```python
from build123d import *

# Parameters (mm, degrees)
SKETCH_1_R      = 1.5
SKETCH_1_W      = 15
SKETCH_1_H      = 18
SKETCH_1_H_2    = 3
EXTRUDE_1_DEPTH = 3
FILLET_1_R      = 5


with BuildPart() as part:
    # 草图1 → 凸台-拉伸1 (new body)
    with BuildSketch(Plane.XY):
        with BuildLine():
            Line((0, 0), (0, 67))
            Line((0, 67), (20, 67))
            Line((20, 67), (22.897896607, 50.56521166))
            ThreePointArc((22.897896607, 50.56521166), (24.147168803, 48.042864005), (26.561036073, 46.595050647))
            ThreePointArc((26.561036073, 46.595050647), (37.908605389, 40.597944156), (45.388192925, 30.167777045))
            ThreePointArc((45.388192925, 30.167777045), (46.877900379, 28.176180142), (49.14284363, 27.148698467))
            Line((49.14284363, 27.148698467), (67, 24))
            Line((67, 24), (67, 0))
            Line((67, 0), (0, 0))
        make_face()
        with Locations((12, 62)):
            Circle(SKETCH_1_R, mode=Mode.SUBTRACT)
        with Locations((12, 42)):
            Circle(SKETCH_1_R, mode=Mode.SUBTRACT)
        with Locations((12, 22)):
            Circle(SKETCH_1_R, mode=Mode.SUBTRACT)
        with Locations(Location((62, 12, 0), (0, 0, 180))):
            Circle(SKETCH_1_R, mode=Mode.SUBTRACT)
        with Locations(Location((42, 12, 0), (0, 0, 180))):
            Circle(SKETCH_1_R, mode=Mode.SUBTRACT)
        with Locations(Location((22, 12, 0), (0, 0, 180))):
            Circle(SKETCH_1_R, mode=Mode.SUBTRACT)
        with Locations((27, 28.5)):
            Rectangle(SKETCH_1_W, SKETCH_1_H, mode=Mode.SUBTRACT)
        with Locations((52, 21)):
            Rectangle(SKETCH_1_W, SKETCH_1_H_2, mode=Mode.SUBTRACT)
    extrude(amount=EXTRUDE_1_DEPTH)

    # 圆角1
    fillet_1_edges = [part.edges().sort_by_distance(p)[0] for p in [
        (0, 0, 1.5),
        (0, 67, 1.5),
        (20, 67, 1.5),
        (67, 24, 1.5),
        (67, 0, 1.5),
    ]]
    fillet(fillet_1_edges, radius=FILLET_1_R)


solid = part.part
```
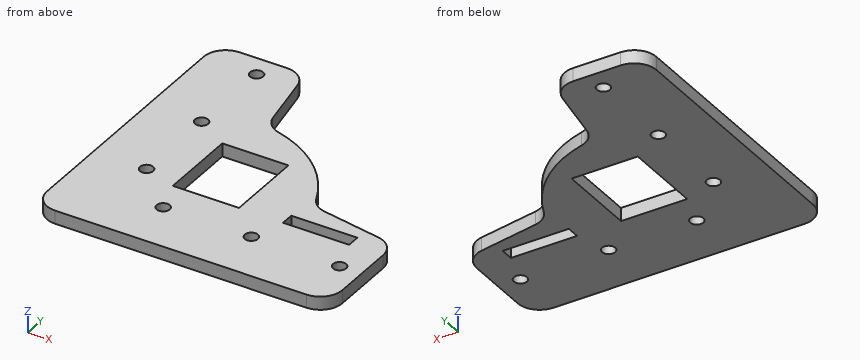
Design review of the part built by this model. Coordinates are the model's own, in mm. Give positions to 0.01 mm unless a question says otherwise; leave off trailing zeros. Order: outer loops, then holes, each group sorted by start corner. A loop starts at its lowest first (then second) coordinate and runs counter-clockwise, first axis right, second up. Notation, with made-up numbers: (77.5, 38.5) - (91.5, 38.5) arc R9 ccw to (91.5, 42.5) - close; hole circle Ø7 at (68.25, 15.5). An arc over 180 degrees is marked (long way). Use a Markdown table: item, result. Add a question column.
(1) Clearance check with flat-ended pins moving along their axes: P1, Ø1.8, axis at x = 42, y = 12, coming from the -Z side; P2, Ø1.5, axis at x = 49, z = 1.5, coming from the +Y side; P3, Ø1, axis at x = 42, z = 1, coming from the +Y side; P4, Ø0.9, axis at y = 28.5, z = 2, coming from the +X side. State where each tip first meets the part, or that it passes through.
(2) Add section C-C on z = 1.65. Give the number of separate pieces and of enclosed holes in the cut face, then the cut area to 3 significant figures.
(3) Wall thickness on probe 1 along X at (y, z) = (12, 1.4); probe 2 along Y at (x, z) = (32.5, 1): over which ranges is each line inside the solid? List them lowest first. Write a range as [from, to].
(4) Add section D-D on x = 24.5. Give the boundary of the cut face in (y, z), then the cut area to 3 significant figures.
(5) Add section A-A on y = 12. Give the boundary of the cut face in (x, z).
Report:
| question | item | result |
|---|---|---|
| 1 | P1 | passes through |
| 1 | P2 | stops at y = 27.39 |
| 1 | P3 | stops at y = 36.82 |
| 1 | P4 | stops at x = 47.04 |
| 2 | separate pieces | 1 |
| 2 | enclosed holes | 8 |
| 2 | area | 2,640 mm² |
| 3 | probe 1 | x = [0, 20.5], [23.5, 40.5], [43.5, 60.5], [63.5, 67] |
| 3 | probe 2 | y = [0, 19.5], [37.5, 44.3] |
| 4 | outline | (0, 0) - (19.5, 0) - (19.5, 3) - (0, 3) - close; (37.5, 0) - (47.7, 0) - (47.7, 3) - (37.5, 3) - close |
| 4 | area | 89.1 mm² |
| 5 | outline | (0, 0) - (20.5, 0) - (20.5, 3) - (0, 3) - close; (23.5, 0) - (40.5, 0) - (40.5, 3) - (23.5, 3) - close; (43.5, 0) - (60.5, 0) - (60.5, 3) - (43.5, 3) - close; (63.5, 0) - (67, 0) - (67, 3) - (63.5, 3) - close |
